from build123d import *

# Parameters (mm, degrees)
SKETCH_1_W          = 100
SKETCH_1_H          = 65
EXTRUDE_1_DEPTH     = 18
SKETCH_2_W          = 55
SKETCH_2_H          = 60
CUT_EXTRUDE_1_DEPTH = 16
SKETCH_3_W          = 15
SKETCH_3_H          = 5
CUT_EXTRUDE_2_DEPTH = 62.743420702
SKETCH_4_W          = 20
SKETCH_4_H          = 56
CUT_EXTRUDE_3_DEPTH = 12
SKETCH_5_W          = 20
SKETCH_5_H          = 40
CUT_EXTRUDE_4_DEPTH = 61.829680256
SKETCH_6_R          = 2
CUT_EXTRUDE_5_DEPTH = 61.829680256
SKETCH_7_R          = 1.5
CUT_EXTRUDE_6_DEPTH = 84.958322994
FILLET_1_R          = 2
FILLET_2_R          = 1
FILLET_3_R          = 4
FILLET_4_R          = 2
FILLET_5_R          = 1


with BuildPart() as part:
    # 草图1 → 凸台-拉伸1 (new body)
    with BuildSketch(Plane.XY):
        Rectangle(SKETCH_1_W, SKETCH_1_H)
    extrude(amount=EXTRUDE_1_DEPTH)

    # 草图2 → 切除-拉伸1 (cut)
    with BuildSketch(Plane.XY.offset(18)):
        Rectangle(SKETCH_2_W, SKETCH_2_H)
    extrude(amount=-CUT_EXTRUDE_1_DEPTH, mode=Mode.SUBTRACT)

    # 草图3 → 切除-拉伸2 (cut, through all)
    with BuildSketch(Plane.XY.offset(2)):
        with Locations((0, -12.5)):
            Rectangle(SKETCH_3_W, SKETCH_3_H)
    extrude(amount=-CUT_EXTRUDE_2_DEPTH, mode=Mode.SUBTRACT)

    # 草图4 → 切除-拉伸3 (cut)
    with BuildSketch(Plane.XY.offset(18)):
        with Locations((40, 0)):
            Rectangle(SKETCH_4_W, SKETCH_4_H)
    cut_extrude_3 = extrude(amount=-CUT_EXTRUDE_3_DEPTH, mode=Mode.SUBTRACT)

    # 草图5 → 切除-拉伸4 (cut, through all)
    with BuildSketch(Plane.XY.offset(6)):
        with Locations((40, 0)):
            Rectangle(SKETCH_5_W, SKETCH_5_H)
    cut_extrude_4 = extrude(amount=-CUT_EXTRUDE_4_DEPTH, mode=Mode.SUBTRACT)

    # 草图6 → 切除-拉伸5 (cut, through all)
    with BuildSketch(Plane.XY.offset(6)):
        with Locations((45, 24)):
            Circle(SKETCH_6_R)
        with Locations((35, 24)):
            Circle(SKETCH_6_R)
        with Locations(Location((35, -24, 0), (0, 0, 180))):
            Circle(SKETCH_6_R)
        with Locations(Location((45, -24, 0), (0, 0, 180))):
            Circle(SKETCH_6_R)
    cut_extrude_5 = extrude(amount=-CUT_EXTRUDE_5_DEPTH, mode=Mode.SUBTRACT)

    # 草图7 → 切除-拉伸6 (cut, through all)
    with BuildSketch(Plane(origin=(0, 32.5, 0), x_dir=(1, 0, 0), z_dir=(0, 1, 0))):
        with Locations(Location((40, -12, 0), (0, 0, 270))):
            Circle(SKETCH_7_R)
    cut_extrude_6 = extrude(amount=-CUT_EXTRUDE_6_DEPTH, mode=Mode.SUBTRACT)

    # 镜向1: 切除-拉伸3, 切除-拉伸4, 切除-拉伸5, 切除-拉伸6 across plane
    add(cut_extrude_3.mirror(Plane(origin=(0, 0, 0), x_dir=(0, 0, 1), z_dir=(1, 0, 0))), mode=Mode.SUBTRACT)
    add(cut_extrude_4.mirror(Plane(origin=(0, 0, 0), x_dir=(0, 0, 1), z_dir=(1, 0, 0))), mode=Mode.SUBTRACT)
    add(cut_extrude_5.mirror(Plane(origin=(0, 0, 0), x_dir=(0, 0, 1), z_dir=(1, 0, 0))), mode=Mode.SUBTRACT)
    add(cut_extrude_6.mirror(Plane(origin=(0, 0, 0), x_dir=(0, 0, 1), z_dir=(1, 0, 0))), mode=Mode.SUBTRACT)

    # 圆角1
    fillet_1_edges = [part.edges().sort_by_distance(p)[0] for p in [
        (27.5, 0, 2),
        (27.5, 30, 10),
        (0, -30, 2),
        (27.5, -30, 10),
        (-27.5, 0, 2),
        (-27.5, -30, 10),
        (0, 30, 2),
        (-27.5, 30, 10),
    ]]
    fillet(fillet_1_edges, radius=FILLET_1_R)

    # 圆角2
    fillet_2_edges = [part.edges().sort_by_distance(p)[0] for p in [
        (7.5, -10, 1),
        (7.5, -15, 1),
        (-7.5, -15, 1),
        (-7.5, -10, 1),
    ]]
    fillet(fillet_2_edges, radius=FILLET_2_R)

    # 圆角3
    fillet_3_edges = [part.edges().sort_by_distance(p)[0] for p in [
        (-50, 30.25, 18),
        (50, -30.25, 18),
        (50, 30.25, 18),
        (-50, -30.25, 18),
    ]]
    fillet(fillet_3_edges, radius=FILLET_3_R)

    # 圆角4
    fillet_4_edges = [part.edges().sort_by_distance(p)[0] for p in [
        (-50, -26.25, 0),
        (-50, 26.25, 0),
        (50, -26.25, 0),
        (50, 26.25, 0),
    ]]
    fillet(fillet_4_edges, radius=FILLET_4_R)

    # 圆角5
    fillet_5_edges = [part.edges().sort_by_distance(p)[0] for p in [
        (-30, 28, 12),
        (-30, -28, 12),
        (-39, -20, 0),
        (-50, 20, 4),
        (-39, 20, 0),
        (-49.414213562, 20, 0.585786438),
        (39, 20, 0),
        (-50, -20, 4),
        (-49.414213562, -20, 0.585786438),
        (50, -20, 4),
        (49.414213562, -20, 0.585786438),
        (50, 20, 4),
        (49.414213562, 20, 0.585786438),
        (30, 28, 12),
        (30, -28, 12),
        (39, -20, 0),
    ]]
    fillet(fillet_5_edges, radius=FILLET_5_R)


solid = part.part
Design review of the part built by this model. Coordinates are the model's own, in mm. A direction names the side the tool comes from. Round coordinates to 2 decimals unless told otherwise and drop trailing zeros. Loops run counter-clockwise (first coordinate to the right, second up) from the corner with the lowest first, then second, coordinate; pieces in that order, holes last. Notation, with made-up numbers: M 78.25,8 L 127.25,8 A27 cw 127.25,24 Z; hole C 9.5,38.5 d8. An arc over 180 degrees is marked long. Answer as a JSON object with one key per item and string values.
Item 1: Machinability: for faces 1 (the flat face through (7.5, -13, 1)), 2 (the flat face through (-39, 20, 4)), 3 (the cylindrical face through (0.36, -29.43, 2.6)), 4 (the flat face through (39, 20, 4)), which of the approach directions +Z, -Z, +X, -X, +Y, -Y give a long, thin tool a straight path to every point of the face, cutting with its end or side? Answer none if there is none.
Answer sheet:
{"face 1": "+Z, -Z", "face 2": "+Z, -Z, -X", "face 3": "+Z", "face 4": "+Z, -Z, +X"}
Item 2: Clearance check with flat-ended pins moving along their axes: P1, Ø12, axis at x = -2.5, y = 12.5, coming from the +Z side; P2, Ø1, axis at y = -12.5, z = 1, coming from the +X side; P3, Ø1.6, axis at y = -12.5, z = 1.5, coming from the -X side; P4, Ø5, axis at x = 40, z = 12, coming from the -Y side. State where each tip first meets the part, or that it passes through.
Answer sheet:
{"P1": "stops at z = 2", "P2": "stops at x = 30", "P3": "stops at x = -30", "P4": "stops at y = -32.5"}
Item 3: We need section D-D on x = 5. Give the boundary of the cut face in (y, z).
Answer sheet:
{"outline": "M -32.5,0 L -15,0 L -15,2 L -28,2 A2 cw -30,4 L -30,18 L -32.5,18 Z; M -10,0 L 32.5,0 L 32.5,18 L 30,18 L 30,4 A2 cw 28,2 L -10,2 Z"}
Item 4: We need section C-C on z = 8.25. Give the boundary of the cut face in (x, y), and give its area (3 significant figures).
Answer sheet:
{"outline": "M -50,-32.5 L 50,-32.5 L 50,-28 L 31,-28 A1 cw 30,-27 L 30,27 A1 cw 31,28 L 50,28 L 50,32.5 L -50,32.5 L -50,28 L -31,28 A1 cw -30,27 L -30,-27 A1 cw -31,-28 L -50,-28 Z; hole M -27.5,-28 A2 ccw -25.5,-30 L 25.5,-30 A2 ccw 27.5,-28 L 27.5,28 A2 ccw 25.5,30 L -25.5,30 A2 ccw -27.5,28 Z", "area": "964 mm^2"}
Item 5: We need section A-A on x = -45. Give the boundary of the cut face in (y, z).
Answer sheet:
{"outline": "M -32.5,0 L -26,0 L -26,6 L -28,6 L -28,18 L -32.5,18 Z; M -22,0 L -21,0 A1 ccw -20,1 L -20,6 L -22,6 Z; M 20,1 A1 ccw 21,0 L 22,0 L 22,6 L 20,6 Z; M 26,0 L 32.5,0 L 32.5,18 L 28,18 L 28,6 L 26,6 Z"}
Item 6: The part is to be moulded in two halves that separate along X. For faces 5 (the flat face through (-38, 28, 12)), 6 (the cylindrical face through (38.536, 30.282, 11.675)), 7 (the flat face through (50, 29, 7)), say which applies: pulls with the +X half, pulls with the -X half, needs draft (parallel to the pull), parting line crosses it, or undercut.
Answer sheet:
{"face 5": "needs draft", "face 6": "undercut", "face 7": "pulls with the +X half"}
Item 7: We need section B-B on y = -24. State how many separate pieces and enclosed holes the cut face has, and give its area (3 significant figures).
Answer sheet:
{"separate pieces": "5", "enclosed holes": "0", "area": "344 mm^2"}
Item 8: Wall thickness on L1, parallel to Y at x = 35, z = 2.7; L2, parallel to X at y = 31, z = 12; L3, parallel to Y at x = -24.5, z = 16.5: over which ranges is each line inside the solid? List them lowest first. Write a range as from..to.
Answer sheet:
{"L1": "y = -32.5..-26, -22..-20, 20..22, 26..32.5", "L2": "x = -50..-41.5, -38.5..38.5, 41.5..50", "L3": "y = -32.5..-30, 30..32.5"}
